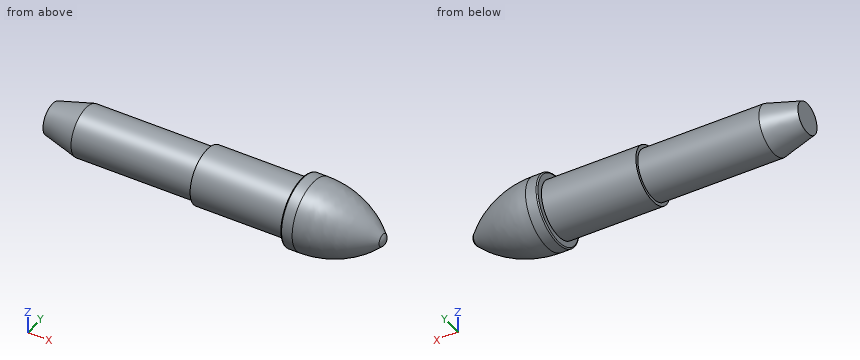
```python
from build123d import *

# Parameters (mm, degrees)
FILLET1_R = 0.1


with BuildPart() as part:
    # Sketch1 → Base-Revolve (revolve)
    with BuildSketch(Plane.XY, mode=Mode.PRIVATE) as base_revolve_sk:
        with BuildLine():
            Line((0, 0), (0, 1.335))
            Line((0, 1.335), (2.836358614, 2.095))
            Line((2.836358614, 2.095), (13.09, 2.095))
            Line((13.09, 2.095), (13.09, 2.375))
            Line((13.09, 2.375), (21.09, 2.375))
            Line((21.09, 2.375), (21.09, 2.955))
            Line((21.09, 2.955), (22.084715758, 2.955))
            ThreePointArc((22.084715758, 2.955), (25.270167636, 2.325954543), (27.977387049, 0.533256881))
            ThreePointArc((27.977387049, 0.533256881), (28.142112811, 0.288928809), (28.2, 0))
            Line((28.2, 0), (0, 0))
        make_face()
    revolve(base_revolve_sk.sketch.rotate(Axis((0, 0, 0), (1, 0, 0)), 90), axis=Axis((0, 0, 0), (1, 0, 0)))

    # Fillet1
    fillet1_edges = [part.edges().sort_by_distance(p)[0] for p in [
        (21.09, 0, -2.955),
    ]]
    fillet(fillet1_edges, radius=FILLET1_R)


solid = part.part
```
Source: CAD feature listing. Evaluate the final solid. Frame: model axes, mm. Round coordinates to 2 decimals unless told otherwise and drop trailing zeros. Order: outer loops, then holes, each group sorted by start corner. A loop starts at its lowest first (then second) coordinate and runs counter-clockwise, first axis right, second up. Notation, with made-up numbers: (-20.75, 72.5) -> (29.25, 72.5) arc R24 ccw to (29.25, 92.5) -> close; hole circle Ø2 at (-27.5, 24). An arc over 180 degrees is marked (long way). One line per item, written item: value. Start each with the question number.
Q1. Section query A-A (x = 20.75). Return the cut outline in (y, z) (3 decimals).
Q2. Material intervals for probe 1 along Z at (x, y) = (17.5, 0.15); probe 2 along Z at (x, y) = (5.25, -0.1); probe 3 along Y at (x, z) = (1, -0.5), sorted ascending.
Q3. Pin query (flat end, axial travel): pin 1 (1.5 mm diameter, centred on x = 12, y = -2, fed in from -Z); pin 2 (1 mm diameter, centred on x = 20, z = 1.5, fed in from -Y); pin 3 (1.5 mm diameter, centred on x = 17.5, y = 1, fed in from +Z). Return the tip coordinate at first contact, or that it passes through.
Findings below:
1. outline: circle Ø4.75 at (0, 0)
2. probe 1: -2.37 to 2.37
2. probe 2: -2.09 to 2.09
2. probe 3: -1.52 to 1.52
3. pin 1: z = -1.68
3. pin 2: y = -2.15
3. pin 3: z = 2.36
